Source: three-view drawing plus pictorial views. Frame: mm from the lowest corner of the part. A direction names the side the tool comes from. Round coordinates to 2 decimals unless told otherwise and drop trailing zeros. Order: outer loops, then holes, each group sorted by start corner. A loop starts at its lowest first (then second) coordinate and runs counter-clockwise, first axis right, second up. Notation, with made-up numbers: (41, 80.5) - (87, 80.5) arc R20 ccw to (87, 118.5) - close; hole circle Ø10 at (57, -37.75). An arc over 180 degrees is marked (long way). One line per item, written item: value. Start each with the question number.
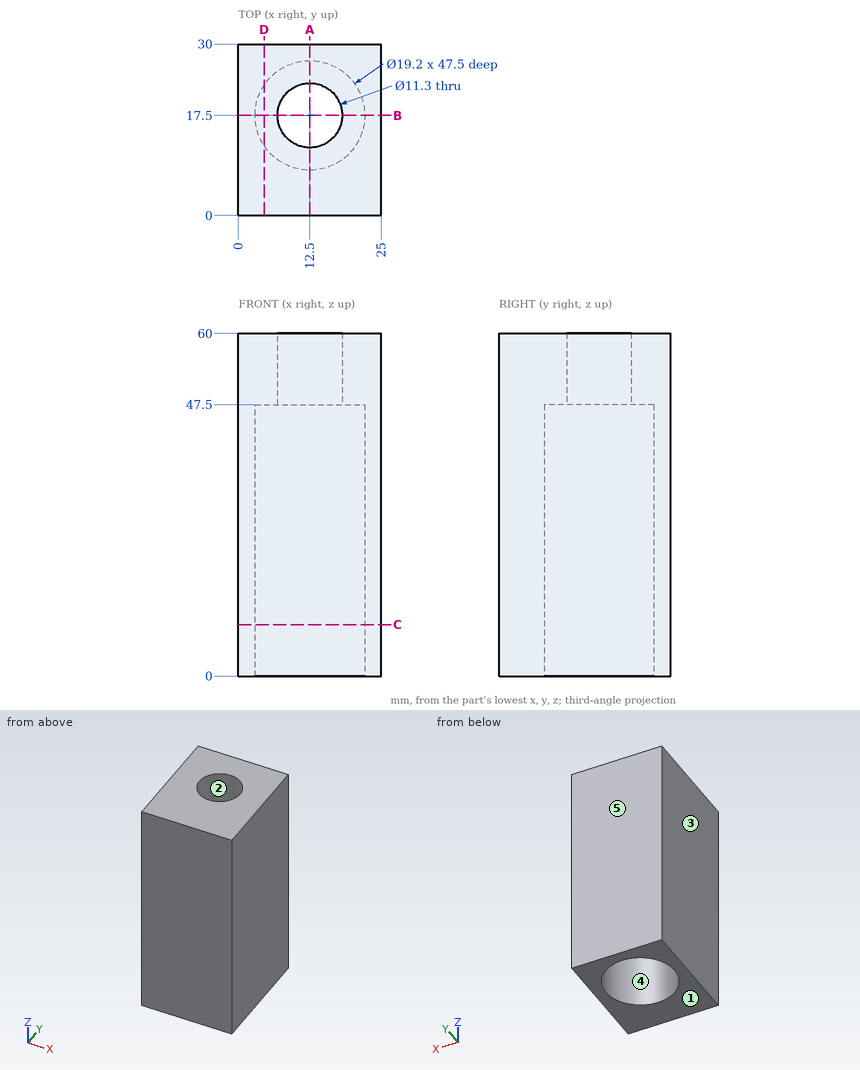
Item 1: Line query: L1, parallel to Y at x = 12.5, z = 54.75; L2, parallel to Y at x = 12, z = 13.5; L3, parallel to X at y = 24, z = 7. Output: solid intervals per line, ascending.
Item 2: Section query C-C on z = 9. Return loops of the section in (x, y).
Item 3: First-contact query: pin 1 Ø4 at (x, y) = (13, 24) entering from -Z. Flat tip, straight axial feed; report the tip coordinate or a pass-through.
Item 4: Section query A-A on x = 12.5. Return loops of the section in (y, z), and give its area (3 significant figures).
Item 5: Section query B-B on y = 17.5. Return loops of the section in (x, z), and give its area (3 significant figures).
Item 6: Section query D-D on x = 4.5. Return loops of the section in (y, z), and give its area (3 significant figures).
Item 7: Pull-direction query (X, two-part tool) for the marked faces 1, 2 and 3; classes: released by +X, released by -X, zero draft, split by the parting line, or undercut.
Item 8: Reachability of the marked faces 4 and 5 from +Z, -Z, +X, -X, +Y, -Y: full face, straight path, thin tool, end or side. Return the list, or none.
Geometry results:
1. L1: y = 0 to 11.85, 23.15 to 30
1. L2: y = 0 to 7.91, 27.09 to 30
1. L3: x = 0 to 5.44, 19.56 to 25
2. outline: (0, 0) - (25, 0) - (25, 30) - (0, 30) - close; hole circle Ø19.2 at (12.5, 17.5)
3. pin 1: stops at z = 47.5
4. outline: (0, 0) - (7.9, 0) - (7.9, 47.5) - (11.85, 47.5) - (11.85, 60) - (0, 60) - close; (23.15, 47.5) - (27.1, 47.5) - (27.1, 0) - (30, 0) - (30, 60) - (23.15, 60) - close
4. area: 747 mm^2
5. outline: (0, 0) - (2.9, 0) - (2.9, 47.5) - (6.85, 47.5) - (6.85, 60) - (0, 60) - close; (18.15, 47.5) - (22.1, 47.5) - (22.1, 0) - (25, 0) - (25, 60) - (18.15, 60) - close
5. area: 447 mm^2
6. outline: (0, 0) - (12.19, 0) - (12.19, 47.5) - (22.81, 47.5) - (22.81, 0) - (30, 0) - (30, 60) - (0, 60) - close
6. area: 1,300 mm^2
7. face 1: zero draft
7. face 2: undercut
7. face 3: released by -X
8. face 4: -Z
8. face 5: +Z, -Z, +X, -X, +Y
